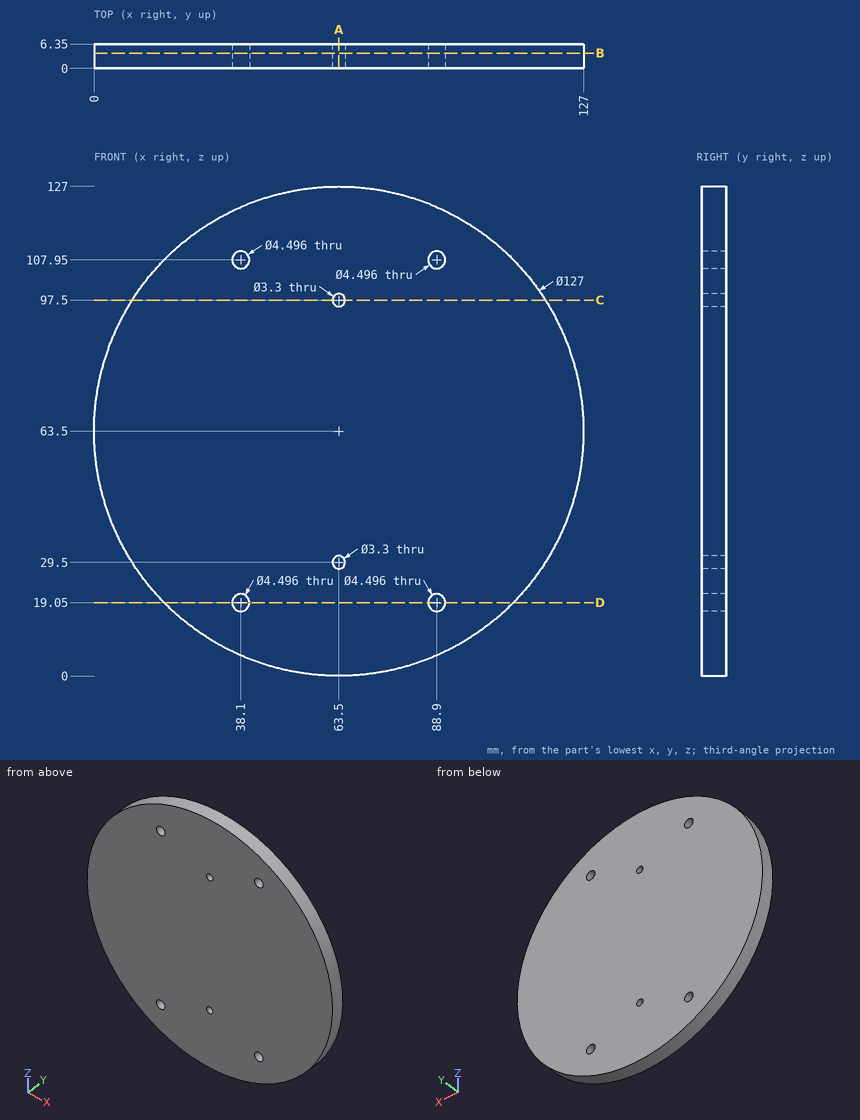
Answer from the drawing. Dimensions are ordinates in mm from the lowest x, y and z of the part. Round coordinates to 2 decimals unless told otherwise and drop trailing zeros. Order: outer loops, then holes, each group sorted by start corner. A loop starts at its lowest first (then second) coordinate and runs counter-clockwise, first axis right, second up.
1) The part is cut by section A-A on x = 63.5. Write down the section's boundary in (y, z).
2) The part is cut by section C-C on z = 97.5. Write down the section's boundary in (x, y), plus the area to 3 significant figures.
3) Straight lines are drawn through the part: L1, parallel to Z at x = 38.1, y = 2.5; L2, parallel to X at y = 2.5, z = 107.95; L3, parallel to X at y = 6, z = 110 (1 decimal). For each, find the intervals that lie inside material, in ascending order.
4) The part is cut by section D-D on z = 19.05. Write down the section's boundary in (x, y), plus the area to 3 significant figures.
5) The part is cut by section B-B on y = 4. Write down the section's boundary in (x, z), plus the area to 3 significant figures.
6) Flat-ended cylindrical pins translate along their axes: pin 1 (4 mm diameter, centred on x = 38.1, z = 19.05, fed in from -Y); pin 2 (2 mm diameter, centred on x = 91, y = 5, fed in from -Z); pin 3 (3 mm diameter, centred on y = 4.5, z = 83, fed in from -X) (1 decimal); pin 4 (2 mm diameter, centred on x = 108, y = 4, fed in from -Z). Find the tip coordinate at first contact, or state that the pin passes through.
Resolved:
1. outline: (0, 0) - (6.35, 0) - (6.35, 27.85) - (0, 27.85) - close; (0, 31.15) - (6.35, 31.15) - (6.35, 95.85) - (0, 95.85) - close; (0, 99.15) - (6.35, 99.15) - (6.35, 127) - (0, 127) - close
2. outline: (9.87, 0) - (61.85, 0) - (61.85, 6.35) - (9.87, 6.35) - close; (65.15, 0) - (117.13, 0) - (117.13, 6.35) - (65.15, 6.35) - close
2. area: 660 mm2
3. L1: z = 5.3 to 16.8, 21.3 to 105.7, 110.2 to 121.7
3. L2: x = 18.15 to 35.85, 40.35 to 86.65, 91.15 to 108.85
3. L3: x = 20.3 to 37.2, 39 to 88, 89.8 to 106.7
4. outline: (18.15, 0) - (35.85, 0) - (35.85, 6.35) - (18.15, 6.35) - close; (40.35, 0) - (86.65, 0) - (86.65, 6.35) - (40.35, 6.35) - close; (91.15, 0) - (108.85, 0) - (108.85, 6.35) - (91.15, 6.35) - close
4. area: 519 mm2
5. outline: circle Ø127 at (63.5, 63.5); hole circle Ø4.5 at (38.1, 19.05); hole circle Ø4.5 at (38.1, 107.95); hole circle Ø3.3 at (63.5, 29.5); hole circle Ø3.3 at (63.5, 97.5); hole circle Ø4.5 at (88.9, 19.05); hole circle Ø4.5 at (88.9, 107.95)
5. area: 12,600 mm2
6. pin 1: passes through
6. pin 2: stops at z = 5.79
6. pin 3: stops at x = 2.6
6. pin 4: stops at z = 17.24
